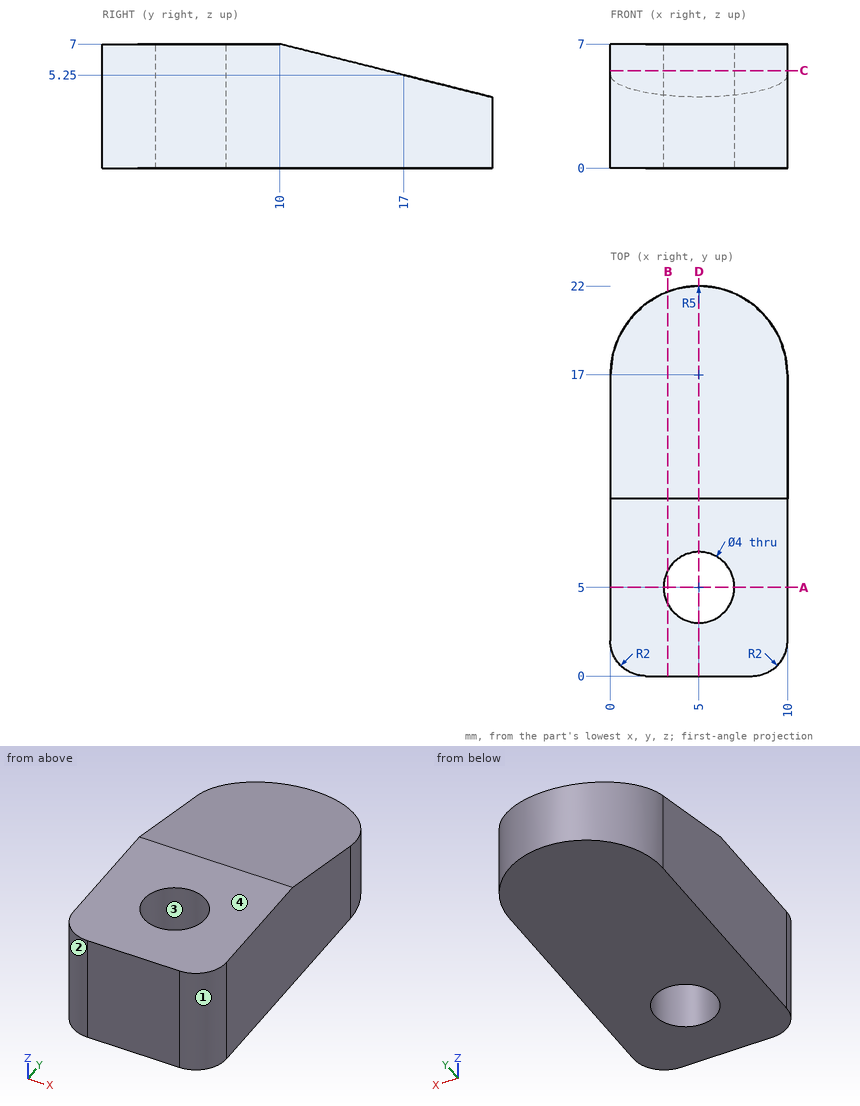
Design review of the part shown in the three views and the two pictorial views. Dimensions are in mm from the part's minimum x, y and z. Round coordinates to 2 decimals unless told otherwise and drop trailing zeros. Loops run counter-clockwise (first coordinate to the right, second up) from the corner with the lowest first, then second, coordinate; pieces in that order, holes last. Notation, with made-up numbers: M -4,69.25 L 37,69.25 A8 cw 37,81.25 Z; hole C -34.75,-3 d11. An arc over 180 degrees is marked long. Write item = value, one per line.
Item 1: Take a section at C-C on z = 5.5. Write out the cut boundary in (x, y).
Return value:
outline = M 0,2 A2 ccw 2,0 L 8,0 A2 ccw 10,2 L 10,16 L 0,16 Z; hole C 5,5 d4
Item 2: Take a section at B-B on x = 3.25. Write out the cut boundary in (y, z).
Return value:
outline = M 0,0 L 4.03,0 L 4.03,7 L 0,7 Z; M 5.97,0 L 21.68,0 L 21.68,4.08 L 10,7 L 5.97,7 Z
Item 3: Take a section at D-D on x = 5. Write out the cut boundary in (y, z), then the cut area to 3 significant figures.
Return value:
outline = M 0,0 L 3,0 L 3,7 L 0,7 Z; M 7,0 L 22,0 L 22,4 L 10,7 L 7,7 Z
area = 108 mm2
Item 4: For line 1 (Y direction, x = 5, z = 3.5); line 2 (Z direction, x = 7, y = 17); line 3 (Y direction, x = 6.75, z = 3), list the stretches that pass through material, from the lowest coordinate up. Write a range as [from, to].
Return value:
line_1 = [0, 3], [7, 22]
line_2 = [0, 5.25]
line_3 = [0, 4.03], [5.97, 21.68]
Item 5: Insertion check: P1, Ø6, axis at x = 7, y = 14, coming from the +Z side; P2, Ø2.5, axis at x = 5, y = 5, coming from the +Z side; P3, Ø4, axis at x = 4.5, y = 17.5, coming from the +Z side (3 decimals). Each pin has a flat end and moves straight along its axis. Give the tip position at first contact, or say it passes through.
Return value:
P1 = 6.75
P2 = through
P3 = 5.625
Item 6: The part is to be moulded in two halves that separate along X. For the marked faces 1, 2, 3 and 4, say which applies: released by +X, released by -X, zero draft, split by the parting line, or undercut.
Return value:
face_1 = released by +X
face_2 = released by -X
face_3 = undercut
face_4 = zero draft
Item 7: Take a section at A-A on y = 5. Write out the cut boundary in (x, z), then the cut area to 3 significant figures.
Return value:
outline = M 0,0 L 3,0 L 3,7 L 0,7 Z; M 7,0 L 10,0 L 10,7 L 7,7 Z
area = 42.0 mm2
